```python
from build123d import *

# Parameters (mm, degrees)
F0_W          = 25.4
F0_H          = 25.4
F1_DEPTH      = 38.1
F2_T          = -2.54
F3_W          = 19.05
F3_H          = 12.7
F4_DEPTH      = 25.4
F5_W          = 22.86
F5_H          = 2.071403
F6_DEPTH      = 25.4
F6_DEPTH_BACK = 25.4
F7_W          = 22.86
F7_H          = 1.634075
F8_DEPTH      = 25.4
F8_DEPTH_BACK = 25.4


with BuildPart() as f1:
    # F0 (on Top) → F1 (new body)
    with BuildSketch(Plane.XY):
        Rectangle(F0_W, F0_H)
    extrude(amount=F1_DEPTH)

    # F2
    f2_openings = [f1.faces().sort_by_distance(p)[0] for p in [
        (0, 0, 38.1),
    ]]
    offset(amount=F2_T, openings=f2_openings)

    # F3 (on Top) → F4 (cut)
    with BuildSketch(Plane.XY):
        Rectangle(F3_W, F3_H)
    extrude(amount=F4_DEPTH, mode=Mode.SUBTRACT)

    # F5 (on Right) → F6 (cut, two sides)
    with BuildSketch(Plane.YZ) as f6_sk:
        with Locations((0, 2.593235)):
            Rectangle(F5_W, F5_H)
    extrude(amount=F6_DEPTH, mode=Mode.SUBTRACT)
    extrude(f6_sk.sketch, amount=-F6_DEPTH_BACK, mode=Mode.SUBTRACT)

    # F7 (on Right) → F8 (cut, two sides)
    with BuildSketch(Plane.YZ) as f8_sk:
        with Locations((0, 12.831571)):
            Rectangle(F7_W, F7_H)
    extrude(amount=F8_DEPTH, mode=Mode.SUBTRACT)
    extrude(f8_sk.sketch, amount=-F8_DEPTH_BACK, mode=Mode.SUBTRACT)


solid = f1.part
```
Verification items for the finished model (mm, model axes). A direction names the side the tool comes from. Coordinates: 2 decimals unless noted, no trailing zeros. Loops run counter-clockwise (first coordinate to the right, second up) from the corner with the lowest first, then second, coordinate; pieces in that order, holes last. Notation, with made-up numbers: (-10.75, -10.75) -> (11.25, -10.75) arc R16 cw to (11.25, 11.25) -> close; hole circle Ø9 at (-16.75, -7). An arc over 180 degrees is marked (long way). Put each result on its own line as item: value.
1. Section check D-D, the plane z = 11.5. Record the boundary of the cut face in (x, y), then the cut area to 3 significant figures.
Result set:
outline: (-12.7, -12.7) -> (12.7, -12.7) -> (12.7, 12.7) -> (-12.7, 12.7) -> close; hole (-10.16, -10.16) -> (10.16, -10.16) -> (10.16, 10.16) -> (-10.16, 10.16) -> close
area: 232 mm^2
2. Section check B-B, the plane z = 3. Record the boundary of the cut face in (x, y).
Result set:
outline: (-12.7, -12.7) -> (12.7, -12.7) -> (12.7, -11.43) -> (-12.7, -11.43) -> close; (-12.7, 11.43) -> (12.7, 11.43) -> (12.7, 12.7) -> (-12.7, 12.7) -> close
3. Tool access check on faces 1 (the face through (9.525, 0, 1)), 2 (the face through (0, -10.16, 26)), 3 (the face through (0, 9, 0)), 4 (the face through (0, 12.7, 19)), 5 (the face through (0, -11.43, 13)). Record the directions out of +Z, -Z, +X, -X, +Y, -Y that give a thin tool (end or side, any length) a straight path to the whole face; none if there is none.
Result set:
face 1: +Z, -Z
face 2: +Z
face 3: -Z, +X, -X, +Y, -Y
face 4: +Z, -Z, +X, -X, +Y
face 5: +X, -X
4. Thickness scan on line 1 (Z direction, x = 10.5, y = -2.25); line 2 (X direction, y = -5, z = 27). Record the ranges inside material, lowest first.
Result set:
line 1: z = 0 to 1.56, 3.63 to 12.01, 13.65 to 38.1
line 2: x = -12.7 to -10.16, 10.16 to 12.7
5. Section check C-C, the plane x = 9. Record the boundary of the cut face in (y, z), then the cut area to 3 significant figures.
Result set:
outline: (-12.7, 0) -> (-6.35, 0) -> (-6.35, 1.56) -> (-11.43, 1.56) -> (-11.43, 3.63) -> (-10.16, 3.63) -> (-10.16, 12.01) -> (-11.43, 12.01) -> (-11.43, 13.65) -> (-10.16, 13.65) -> (-10.16, 38.1) -> (-12.7, 38.1) -> close; (6.35, 0) -> (12.7, 0) -> (12.7, 38.1) -> (10.16, 38.1) -> (10.16, 13.65) -> (11.43, 13.65) -> (11.43, 12.01) -> (10.16, 12.01) -> (10.16, 3.63) -> (11.43, 3.63) -> (11.43, 1.56) -> (6.35, 1.56) -> close
area: 196 mm^2
6. Gauge pin test, flat end, axial feed: P1, Ø10, axis at x = 1.5, y = 4.5, coming from the +Z side. Record the tip position at first contact, or that the pin passes through.
Result set:
P1: stops at z = 1.56
7. Section check A-A, the plane y = -3.75. Record the boundary of the cut face in (x, z) (3 decimals), then the cut area to 3 significant figures.
Result set:
outline: (-12.7, 0) -> (-9.525, 0) -> (-9.525, 1.558) -> (-12.7, 1.558) -> close; (-12.7, 3.629) -> (-10.16, 3.629) -> (-10.16, 12.015) -> (-12.7, 12.015) -> close; (-12.7, 13.649) -> (-10.16, 13.649) -> (-10.16, 38.1) -> (-12.7, 38.1) -> close; (9.525, 0) -> (12.7, 0) -> (12.7, 1.558) -> (9.525, 1.558) -> close; (10.16, 3.629) -> (12.7, 3.629) -> (12.7, 12.015) -> (10.16, 12.015) -> close; (10.16, 13.649) -> (12.7, 13.649) -> (12.7, 38.1) -> (10.16, 38.1) -> close
area: 177 mm^2
8. Mould release check, pull along X, two halves, no side actions. Record for faces 6 (the face through (0, -10.16, 8)), 7 (the face through (12.7, 0, 19)), 8 (the face through (0, -11.43, 3)): pulls with the +X half, pulls with the -X half, needs draft (parallel to the pull), parting line crosses it, or undercut.
Result set:
face 6: undercut
face 7: pulls with the +X half
face 8: needs draft
